Work out the finished part from the listing and answer in its coordinate system (mm). Give positions to 0.01 mm unless a question says otherwise; leave off trailing zeros. Order: outer loops, then holes, each group sorted by start corner. A loop starts at its lowest first (then second) coordinate and runs counter-clockwise, first axis right, second up. Notation, with made-up numbers: (-12.75, -36) - (33.25, -36) arc R26 ccw to (33.25, -18) - close; hole circle Ø6 at (86, -16.5). An arc over 180 degrees is marked (long way). Write each question's results on one line, items separated by ' | '.
from build123d import *

# Parameters (mm, degrees)
SKETCH_1_W          = 25
SKETCH_1_H          = 17
SKETCH_1_R          = 6.5
EXTRUDE_1_DEPTH     = 4
SKETCH_2_R          = 1.5
CUT_EXTRUDE_1_DEPTH = 22.476731595


with BuildPart() as part:
    # 草图1 → 凸台-拉伸1 (new, symmetric)
    with BuildSketch(Plane(origin=(0, 0, 0), x_dir=(1, 0, 0), z_dir=(0, 1, 0))):
        Rectangle(SKETCH_1_W, SKETCH_1_H)
        with Locations(Location((0, 0, 0), (0, 0, 270))):
            Circle(SKETCH_1_R, mode=Mode.SUBTRACT)
    extrude(amount=EXTRUDE_1_DEPTH, both=True)

    # 草图2 → 切除-拉伸1 (cut, through all)
    with BuildSketch(Plane(origin=(0, 0, -8.5), x_dir=(-1, 0, 0), z_dir=(0, 0, -1))):
        with Locations((9.5, 0)):
            Circle(SKETCH_2_R)
        with Locations(Location((-9.5, 0, 0), (0, 0, 180))):
            Circle(SKETCH_2_R)
    extrude(amount=-CUT_EXTRUDE_1_DEPTH, mode=Mode.SUBTRACT)


solid = part.part
1. Determine the mould class of faces 1 (the face through (-6, 4, 4)), 2 (the face through (8, 0, 0)), 3 (the face through (0, 0, -8.5)) for opening direction Y: +Y half, -Y half, draft (parallel to the pull), parting line (faces both ways), or undercut.
Answer list:
face 1: +Y half | face 2: undercut | face 3: draft
2. A cutting plane is placed at C-C, the plane x = 0. Write down the section's boundary in (y, z), then the cut area to 3 significant figures.
Answer list:
outline: (-4, -8.5) - (4, -8.5) - (4, -6.5) - (-4, -6.5) - close; (-4, 6.5) - (4, 6.5) - (4, 8.5) - (-4, 8.5) - close | area: 32.0 mm^2
3. A cutting plane is placed at A-A, the plane y = 0. Write down the section's boundary in (x, z).
Answer list:
outline: (-12.5, -8.5) - (-11, -8.5) - (-11, 8.5) - (-12.5, 8.5) - close; (-8, -8.5) - (8, -8.5) - (8, 8.5) - (-8, 8.5) - close; (11, -8.5) - (12.5, -8.5) - (12.5, 8.5) - (11, 8.5) - close; hole circle Ø13 at (0, 0)
4. Straight lines are drawn through the part: line 1 (X direction, y = 2.25, z = 0); line 2 (Z direction, x = -1.5, y = 2.75); line 3 (Z direction, x = 5.25, y = 3.5). For each, find the intervals that lie inside material, in ascending order. Write a range as [from, to].
Answer list:
line 1: [-12.5, -6.5], [6.5, 12.5] | line 2: [-8.5, -6.32], [6.32, 8.5] | line 3: [-8.5, -3.83], [3.83, 8.5]
5. A cutting plane is placed at B-B, the plane z = 0. Write down the section's boundary in (x, y), then the cut area to 3 significant figures.
Answer list:
outline: (-12.5, -4) - (-6.5, -4) - (-6.5, 4) - (-12.5, 4) - close; (6.5, -4) - (12.5, -4) - (12.5, 4) - (6.5, 4) - close; hole circle Ø3 at (-9.5, 0); hole circle Ø3 at (9.5, 0) | area: 81.9 mm^2
6. A cutting plane is placed at D-D, the plane y = 2. Write down the section's boundary in (x, z), then the cut area to 3 significant figures.
Answer list:
outline: (-12.5, -8.5) - (12.5, -8.5) - (12.5, 8.5) - (-12.5, 8.5) - close; hole circle Ø13 at (0, 0) | area: 292 mm^2
7. Given P1, Ø4, axis at x = -9.5, y = 0, coming from the +Z side, flat-ended and moving along its own axis, determine where the tip first touches the part or whether it passes through.
Answer list:
P1: z = 8.5
